from build123d import *

# Parameters (mm, degrees)
FILLET1_R   = 0.2
HEX_2_DEPTH = 1.3


with BuildPart() as part:
    # BodySke → BaseBody (revolve)
    with BuildSketch(Plane.XY):
        with BuildLine():
            Line((10.2, 0), (10.2, 1.61))
            Line((10.2, 1.61), (9.81, 2))
            Line((9.81, 2), (2.2, 2))
            Line((2.2, 2), (2.2, 3.8))
            Line((2.2, 3.8), (1.82, 3.8))
            ThreePointArc((1.82, 3.8), (0.762013659, 2.991755338), (0, 1.9))
            Line((0, 1.9), (0, 0))
            Line((0, 0), (10.2, 0))
        make_face()
    revolve(axis=Axis((0, 0, 0), (1, 0, 0)))

    # Fillet1
    fillet1_edges = [part.edges().sort_by_distance(p)[0] for p in [
        (2.2, -2, 0),
    ]]
    fillet(fillet1_edges, radius=FILLET1_R)

    # Sketch2 → PreBroach (revolve, cut)
    with BuildSketch(Plane.XY):
        Polygon((0, 1.25), (1.3, 1.25), (2.021687836, 0), (0, 0), align=None)
    revolve(axis=Axis((0, 0, 0), (1, 0, 0)), mode=Mode.SUBTRACT)

    # Sketch3 → Hex 2 (cut)
    with BuildSketch(Plane(origin=(0, 0, 0), x_dir=(0, 0, -1), z_dir=(1, 0, 0))):
        Polygon((-1.25, -0.721687836), (-1.25, 0.721687836), (0, 1.443375673), (1.25, 0.721687836), (1.25, -0.721687836), (0, -1.443375673), align=None)
    extrude(amount=HEX_2_DEPTH, mode=Mode.SUBTRACT)


solid = part.part
CAD build for the part. Positions are in the model's coordinates, mm. A direction names the side the tool comes from. Give positions to 0.01 mm unless a question says otherwise; leave off trailing zeros. Write each loop counter-clockwise with the first axis right and the second up, starting at its lowest first coordinate (ties: lowest second). Pieces come first, ordered by that corner, then holes. Notation, with made-up numbers: (89, 75.5) - (117, 75.5) arc R32 cw to (117, 102.5) - close; hole circle Ø4 at (34, 73). An arc over 180 degrees is marked (long way). Put each result on its own line as item: value.
(1) Saw through at A-A (x = 7.25). List the corners of the cut face in (y, z).
Working result:
outline: circle Ø4 at (0, 0)
(2) Saw through at B-B (z = -3). List the corners of the cut face in (x, y).
Working result:
outline: (1.82, -2.33) - (2.2, -2.33) - (2.2, 2.33) - (1.82, 2.33) arc R3.12 ccw to start
(3) Tool access for faces 4 (the cylindrical face through (6, 0, -2)), 5 (the flat face through (10.2, 0, 0)), 6 (the flat face through (1, 0, 1.25)): list every direction of +Z, -Z, +X, -X, +Y, -Y with a clear straight run to the whole face (end or side of a thin tool).
Working result:
face 4: +X
face 5: +Z, -Z, +X, +Y, -Y
face 6: -X
(4) Saw through at C-C (y = 2.5). List the corners of the cut face in (x, z).
Working result:
outline: (1.82, -2.86) - (2.2, -2.86) - (2.2, 2.86) - (1.82, 2.86) arc R3.53 ccw to start
(5) Drop flat-ended pins along their axis: pin 1 Ø1 at (x, y) = (5.5, 0) entering from -Z; pin 2 Ø0.6 at (x, y) = (1, 0) entering from +Z. Give the stop position or say it passes through.
Working result:
pin 1: z = -2
pin 2: z = 3.47
(6) Pull direction Y, two halves, no side cores. Call faces 1 (the flat face through (2.2, -2, -2)), 2 (the flat face through (1, 0, -1.25)), 3 (the cylindrical face through (2.007, -3.796, 0.167)): released by +Y, released by -Y, zero draft, split by the parting line, or undercut.
Working result:
face 1: zero draft
face 2: undercut
face 3: split by the parting line
(7) Wall check: L1, parallel to Z at x = 9.25, y = 0; L2, parallel to Y at x = 0.75, z = -0.25; L3, parallel to Z at x = 9, y = -1. Give the ranges that are in metal, low to high.
Working result:
L1: -2 to 2
L2: -2.97 to -1.3, 1.3 to 2.97
L3: -1.73 to 1.73
